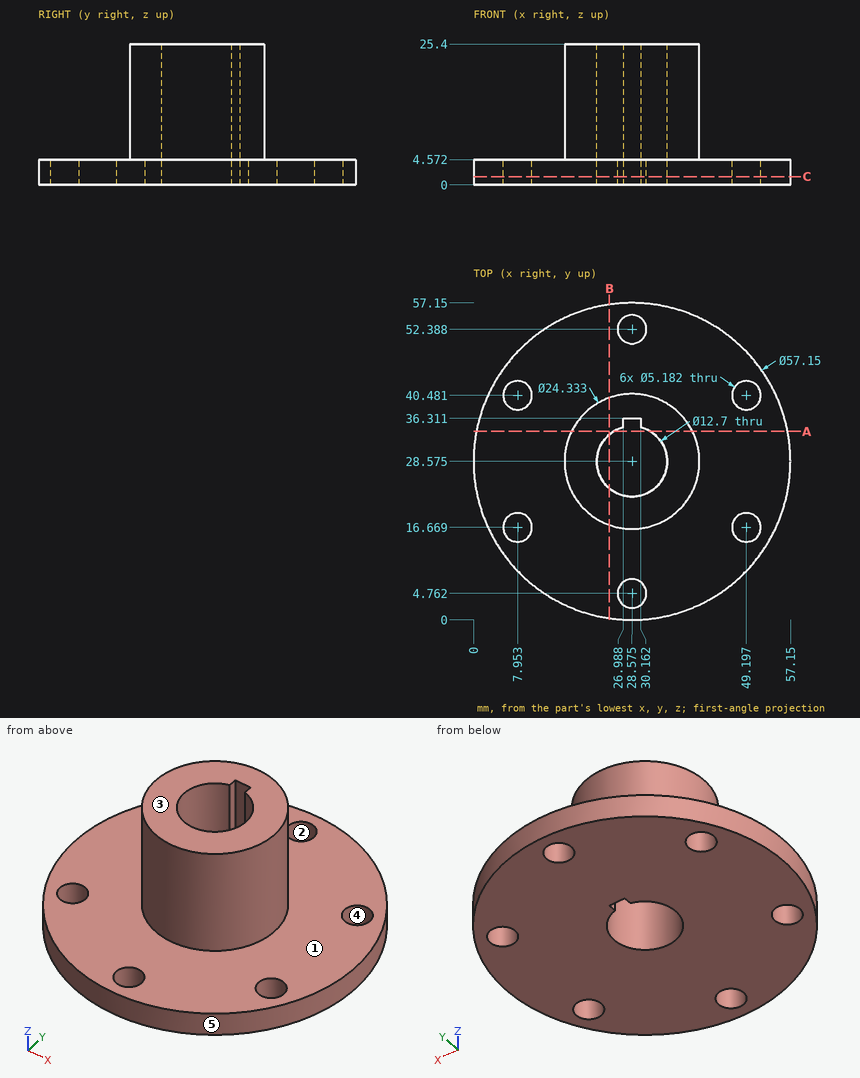
Design review of the part shown in the three views and the two pictorial views. Dimensions are in mm from the part's minimum x, y and z. A direction names the side the tool comes from. Round coordinates to 2 decimals unless told otherwise and drop trailing zeros. Write each loop counter-clockwise with the first axis right and the second up, starting at its lowest first coordinate (ties: lowest second). Pieces come first, ordered by that corner, then holes. Notation, with made-up numbers: (81, 16) - (92, 16) arc R22 cw to (92, 25) - close; hole circle Ø7 at (9, 42). An arc over 180 degrees is marked (long way). Answer as CSV lines item,"result". Start each with the question number.
(1) Machinability: for the marked faces 1 and 2, which of the approach directions +Z, -Z, +X, -X, +Y, -Y give a long, thin tool a straight path to every point of the face, cutting with its end or side? Answer none if there is none.
(2) For pin 1 (0.5 mm diameter, centred on y = 35.5, z = 10.5, fed in from -X); pin 2 (8.5 mm diameter, centred on x = 28.58, y = 4.76, fed in from +Z); pin 3 (4 mm diameter, centred on x = 49.2, y = 40.48, fed in from +Z); pin 4 (3 mm diameter, centred on x = 35, z = 22.5, fed in from +Y), all flat-tipped, find the tip position at first contact; note any pin that passes through.
(3) Add section B-B, the plane x = 24.5. State the section outline as (y, z) points (1 decimal).
(4) Mouldability with a two-part tool opening along Y and no side actions: class the marked faces 3, 4 and 5 as +Y half, -Y half, draft (parallel to the pull), parting line (faces both ways), or undercut.
(5) For line 1 (Z direction, x = 29, y = 46); line 2 (X direction, y = 26, z = 23) (1 decimal); line 3 (X direction, y = 29.5, z = 13), list the stretches that pass through material, from the lowest coordinate up.
(6) Add section A-A, the plane y = 34. State the section outline as (x, z) points (1 decimal).
(7) Add section C-C, the plane z = 1.5. State how many separate pieces and enclosed holes the cut face has, plus the area to 3 significant figures.
From the geometry:
1,face 1,"+Z"
1,face 2,"+Z, -Z"
2,pin 1,"stops at x = 18.4"
2,pin 2,"stops at z = 4.57"
2,pin 3,"passes through"
2,pin 4,"stops at y = 39.7"
3,outline,"(0.3, 0) - (23.7, 0) - (23.7, 25.4) - (17.1, 25.4) - (17.1, 4.6) - (0.3, 4.6) - close; (33.4, 0) - (56.9, 0) - (56.9, 4.6) - (40, 4.6) - (40, 25.4) - (33.4, 25.4) - close"
4,face 3,"draft"
4,face 4,"undercut"
4,face 5,"parting line"
5,line 1,"z = 0 to 4.57"
5,line 2,"x = 16.7 to 22.8, 34.4 to 40.5"
5,line 3,"x = 16.44 to 22.29, 34.86 to 40.71"
6,outline,"(0.5, 0) - (25.3, 0) - (25.3, 25.4) - (17.7, 25.4) - (17.7, 4.6) - (0.5, 4.6) - close; (31.9, 0) - (56.6, 0) - (56.6, 4.6) - (39.5, 4.6) - (39.5, 25.4) - (31.9, 25.4) - close"
7,separate pieces,"1"
7,enclosed holes,"7"
7,area,"2,310 mm²"
